CAD build for the part. Positions are in the model's coordinates, mm. Face numbers are marked on the shaded views. Coordinates: 2 decimals unless noted, no trailing zeros. Order: outer loops, then holes, each group sorted by start corner. A loop starts at its lowest first (then second) coordinate and runs counter-clockwise, first axis right, second up. Notation, with made-up numbers: M 18.25,18.25 L 52.25,18.25 A24 ccw 52.25,55.25 Z; hole C 57.25,11.5 d5. An arc over 180 degrees is marked long. Write item = value, one per line.
from build123d import *

# Parameters (mm, degrees)
F1_DEPTH = 20
F3_DEPTH = 131.803615
F5_DEPTH = 131.803615
F6_W     = 5
F6_H     = 20
F7_DEPTH = 25


with BuildPart() as f1:
    # F0 (on Top) → F1 (new body)
    with BuildSketch(Plane.XY):
        with BuildLine():
            Line((-368.272997, -290), (-368.272997, -300))
            ThreePointArc((-368.272997, -300), (0, -475), (368.272997, -300))
            Line((368.272997, -300), (368.272997, -290))
            Line((368.272997, -290), (-368.272997, -290))
        make_face()
    extrude(amount=F1_DEPTH)

    # F2 (on face) → F3 (join)
    with BuildSketch(Plane.YZ.offset(368.272997)):
        with BuildLine():
            Line((-300, 20), (-300, 5))
            ThreePointArc((-300, 5), (-295, 0), (-290, 5))
            Line((-290, 5), (-290, 20))
            Line((-290, 20), (-300, 20))
        make_face()
    extrude(amount=F3_DEPTH)

    # F4 (on face) → F5 (join)
    with BuildSketch(Plane(origin=(-368.272997, 0, 0), x_dir=(0, -1, 0), z_dir=(-1, 0, 0))):
        with BuildLine():
            Line((290, 20), (290, 5))
            ThreePointArc((290, 5), (291.464466, 1.464466), (295, 0))
            ThreePointArc((295, 0), (298.535534, 1.464466), (300, 5))
            Line((300, 5), (300, 20))
            Line((300, 20), (290, 20))
        make_face()
    extrude(amount=F5_DEPTH)

    # F6 (on face) → F7 (join)
    with BuildSketch(Plane.XY.offset(20)):
        Polygon((-368.272997, -290), (-405.772997, -290), (-405.772997, -300), (-400.772997, -300), (-368.272997, -300), align=None)
        with Locations((-403.272997, -310)):
            Rectangle(F6_W, F6_H)
        Polygon((405.772997, -290), (368.272997, -290), (368.272997, -300), (400.772997, -300), (405.772997, -300), align=None)
        with Locations((403.272997, -310)):
            Rectangle(F6_W, F6_H)
    extrude(amount=F7_DEPTH)


solid = f1.part
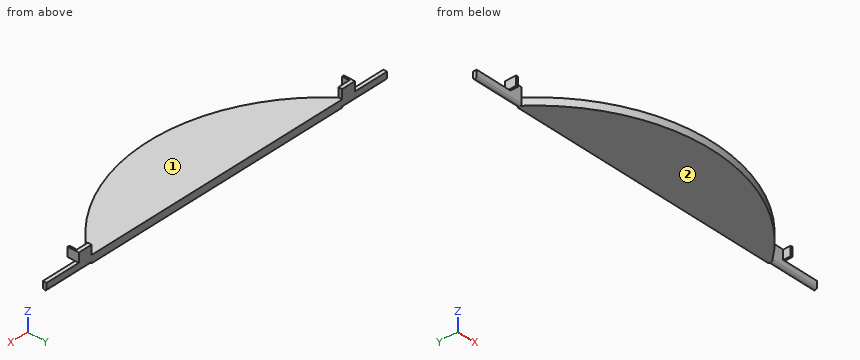
(1) Slice it at C-C, the plane x = 114. Write the cut outline in (y, z), then the cut area to 3 significant figures.
Evaluation:
outline = M -461.12,0 L -290,0 L -290,20 L -461.12,20 Z
area = 3,420 mm²
(2) Pull direction X, two halves, no side cores. Call the marked faces 1 and 2: +X half, -X half, draft (parallel to the pull), parting line (faces both ways), or undercut.
Evaluation:
face_1 = undercut
face_2 = draft
(3) Slice it at A-A, the plane x = -430.5. Write the cut outline in (y, z).
Evaluation:
outline = M -300,5 A5 ccw -290,5 L -290,20 L -300,20 Z
(4) Wall check: line 1 (X direction, y = -302.5, z = 40); line 2 (Z direction, x = 193, y = -338.5); line 3 (Y direction, x = 307, z = 8). Give the ranges that are in metal, low to high. Write a range as from..to.
Evaluation:
line_1 = -405.77..-400.77, 400.77..405.77
line_2 = 0..20
line_3 = -362.46..-290
(5) Pin check, flat tips, straight feed: pin 1 Ø1.5 at (x, z) = (390.5, 22.5) entering from -Y; pin 2 Ø3 at (y, z) = (-318.5, 17.5) entering from -X; pin 3 Ø1.5 at (x, y) = (403, -306) entering from -Z; pin 4 Ø1 at (x, y) = (101.5, -405) entering from -Z. Stop position of each tip, or through.
Evaluation:
pin_1 = -300
pin_2 = -353.75
pin_3 = 20
pin_4 = 0
(6) Slice it at B-B, the plane y = -408. Write the cut outline in (x, z), then the cut area to 3 significant figures.
Evaluation:
outline = M -243.23,0 L 243.23,0 L 243.23,20 L -243.23,20 Z
area = 9,730 mm²
